Verification items for this drawing (mm, ordinates from the low corner). Round coordinates to 2 decimals unless told otherwise and drop trailing zeros. Write each loop counter-clockwise with the first axis right and the second up, starting at its lowest first coordinate (ties: lowest second). Pieces come first, ordered by that corner, then holes. Notation, with made-up numbers: (-16, 13.5) -> (19, 13.5) arc R10 ccw to (19, 27.5) -> close; hole circle Ø8 at (80.25, 4.5). An arc over 180 degrees is marked (long way). One line per item, written item: value.
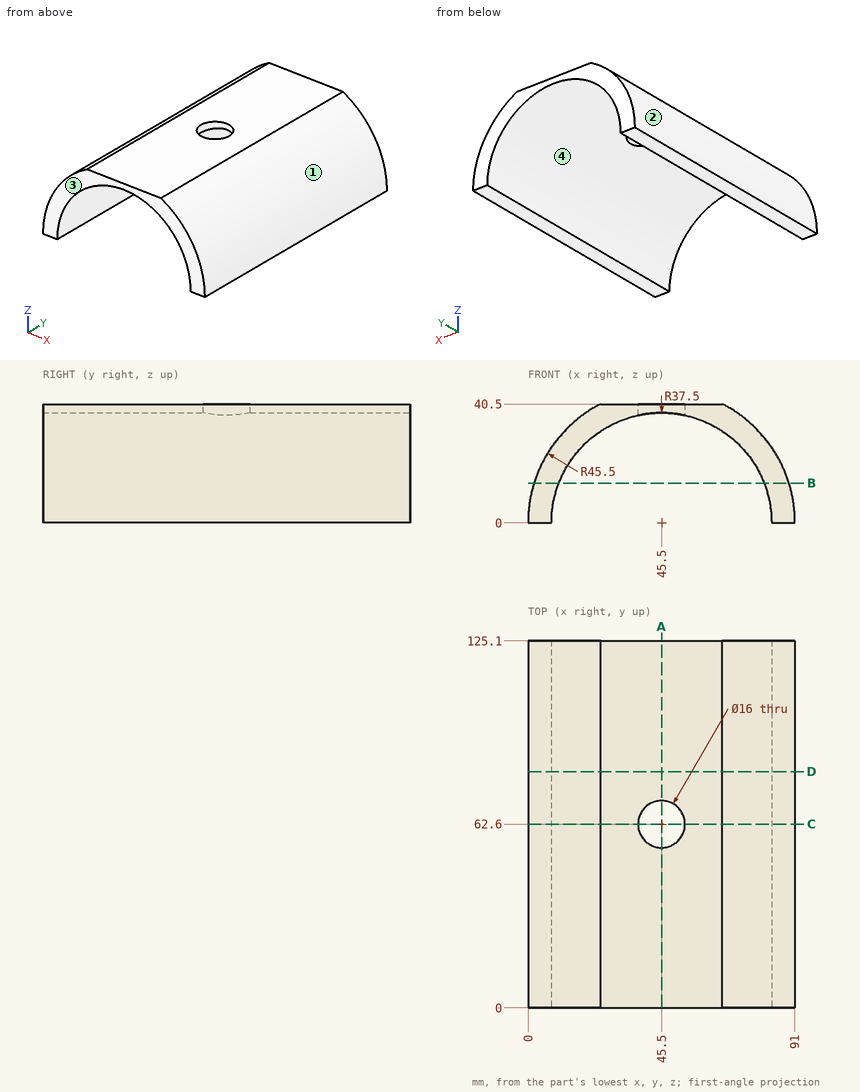
Item 1: Material ranges on line 1 along Y through (x, z) = (45.5, 39.2); line 2 along Z through (x, y) = (45.5, 12); line 3 along X through (y, z) = (5, 29), recorded low to high.
Result set:
line 1: 0 to 54.6, 70.6 to 125.1
line 2: 37.5 to 40.5
line 3: 10.44 to 21.73, 69.27 to 80.56
Item 2: Sectioned sample at C-C (y = 62.6). Enter the section's corners in (x, z).
Result set:
outline: (0, 0) -> (8, 0) arc R37.5 cw to (37.5, 36.64) -> (37.5, 40.5) -> (24.76, 40.5) arc R45.5 ccw to start; (53.5, 36.64) arc R37.5 cw to (83, 0) -> (91, 0) arc R45.5 ccw to (66.24, 40.5) -> (53.5, 40.5) -> close
Item 3: Sectioned sample at D-D (y = 80.5). Enter the section's corners in (x, z).
Result set:
outline: (0, 0) -> (8, 0) arc R37.5 cw to (83, 0) -> (91, 0) arc R45.5 ccw to (66.24, 40.5) -> (24.76, 40.5) arc R45.5 ccw to start
Item 4: Depth check by flat-ended pin: pin 1 (5 mm diameter, centred on y = 26.5, z = 16.5, fed in from +X); pin 2 (3 mm diameter, centred on y = 32, z = 6, fed in from +X); pin 3 (1 mm diameter, centred on x = 30, z = 33.5, fed in from -Y); pin 4 (10 mm diameter, centred on y = 16, z = 33.5, fed in from -X). Enter the tip coordinate at first touch or a pass-through.
Result set:
pin 1: x = 88.79
pin 2: x = 90.78
pin 3: through
pin 4: x = 10.03
Item 5: Sectioned sample at A-A (x = 45.5). Enter the section's corners in (y, z), then the cut area to 3 significant figures.
Result set:
outline: (0, 37.5) -> (54.6, 37.5) -> (54.6, 40.5) -> (0, 40.5) -> close; (70.6, 37.5) -> (125.1, 37.5) -> (125.1, 40.5) -> (70.6, 40.5) -> close
area: 327 mm^2
Item 6: Sectioned sample at B-B (z = 13.5). Enter the section's corners in (x, y).
Result set:
outline: (2.05, 0) -> (10.51, 0) -> (10.51, 125.1) -> (2.05, 125.1) -> close; (80.49, 0) -> (88.95, 0) -> (88.95, 125.1) -> (80.49, 125.1) -> close
Item 7: Release check for a two-part mould opening along X. For the marked faces 1, 2, 3 and 4 record: pulls with the +X half, pulls with the -X half, needs draft (parallel to the pull), parting line crosses it, or undercut.
Result set:
face 1: pulls with the +X half
face 2: pulls with the -X half
face 3: needs draft
face 4: undercut
